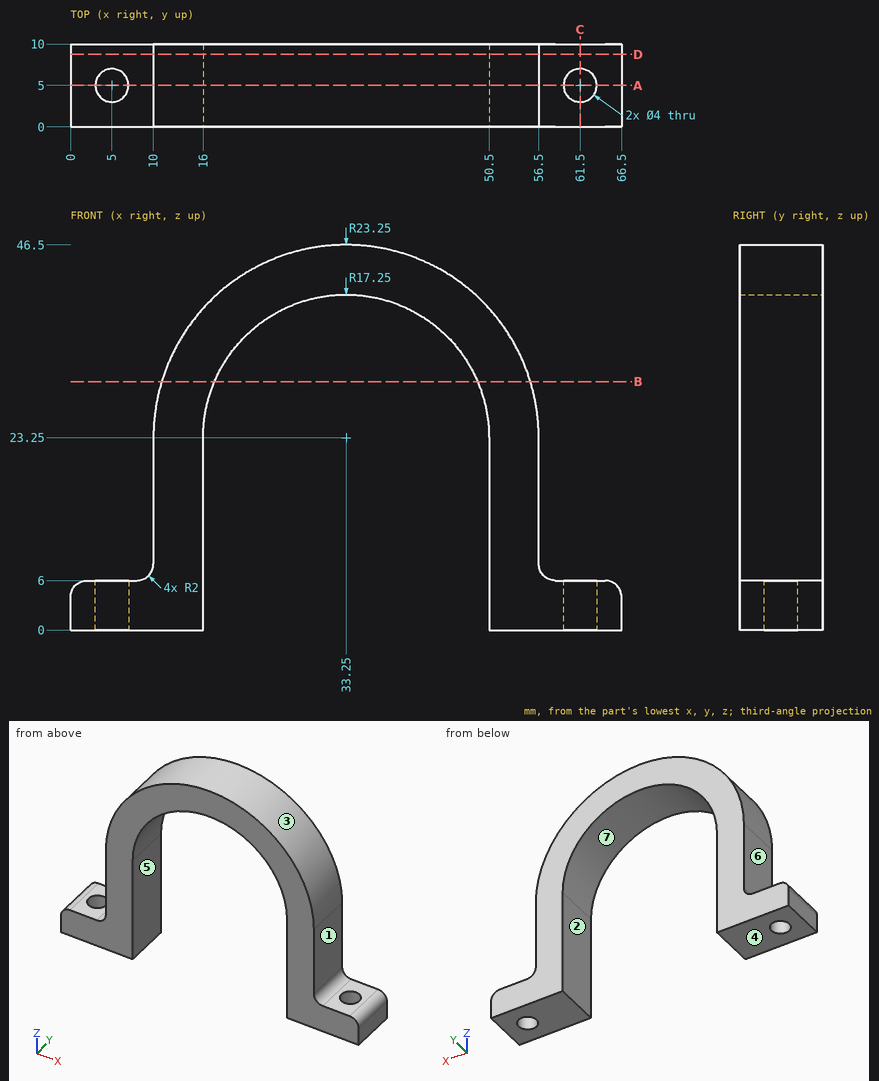
Verification items for this drawing (mm, ordinates from the low corner). A direction names the side the tool comes from. Coordinates: 2 decimals unless noted, no trailing zeros. Loops run counter-clockwise (first coordinate to the right, second up) from the corner with the lowest first, then second, coordinate; pieces in that order, holes last. Notation, with made-up numbers: (78, 15.25) - (118, 15.25) arc R12 ccw to (118, 26.25) - close; hole circle Ø5 at (3, 78.25). An arc over 180 degrees is marked (long way). Answer as a JSON object with one key per item and string values.
(1) Cross-section at A-A, the plane y = 5. Record the boundary of the cut face in (x, z), then the cut area to 3 significant figures.
Response:
{"outline": "(0, 0) - (3, 0) - (3, 6) - (2, 6) arc R2 ccw to (0, 4) - close; (7, 0) - (16, 0) - (16, 23.25) arc R17.25 cw to (50.5, 23.25) - (50.5, 0) - (59.5, 0) - (59.5, 6) - (58.5, 6) arc R2 cw to (56.5, 8) - (56.5, 23.25) arc R23.25 ccw to (10, 23.25) - (10, 8) arc R2 cw to (8, 6) - (7, 6) - close; (63.5, 0) - (66.5, 0) - (66.5, 4) arc R2 ccw to (64.5, 6) - (63.5, 6) - close", "area": "733 mm²"}
(2) Cross-section at D-D, the plane y = 8.75. Record the boundary of the cut face in (x, z).
Response:
{"outline": "(0, 0) - (16, 0) - (16, 23.25) arc R17.25 cw to (50.5, 23.25) - (50.5, 0) - (66.5, 0) - (66.5, 4) arc R2 ccw to (64.5, 6) - (58.5, 6) arc R2 cw to (56.5, 8) - (56.5, 23.25) arc R23.25 ccw to (10, 23.25) - (10, 8) arc R2 cw to (8, 6) - (2, 6) arc R2 ccw to (0, 4) - close"}
(3) Mould release check, pull along X, two halves, no side actions. Record for the marked faces 4, 5, 6 and 7: pulls with the +X half, pulls with the -X half, needs draft (parallel to the pull), parting line crosses it, or undercut.
Response:
{"face 4": "needs draft", "face 5": "undercut", "face 6": "pulls with the -X half", "face 7": "undercut"}
(4) Access from +Z, -Z, +X, -X, +Y, -Y to the whole of each face (thin tool, end or side, straight path). Record for the marked faces 1, 2 and 3.
Response:
{"face 1": "+Z, +X, +Y, -Y", "face 2": "-Z, +Y, -Y", "face 3": "+Z, +Y, -Y"}
(5) Cross-section at C-C, the plane x = 61.5. Record the boundary of the cut face in (y, z), then the cut area to 3 significant figures.
Response:
{"outline": "(0, 0) - (3, 0) - (3, 6) - (0, 6) - close; (7, 0) - (10, 0) - (10, 6) - (7, 6) - close", "area": "36.0 mm²"}
(6) Cross-section at B-B, the plane z = 30. Record the boundary of the cut face in (x, y), then the cut area to 3 significant figures.
Response:
{"outline": "(11, 0) - (17.38, 0) - (17.38, 10) - (11, 10) - close; (49.12, 0) - (55.5, 0) - (55.5, 10) - (49.12, 10) - close", "area": "127 mm²"}
(7) Go/stop test with flat-tipped pins: pin 1 Ø2 at (x, y) = (31, 6.5) entering from +Z; pin 2 Ø5 at (y, z) = (7, 16.5) entering from -X; pin 3 Ø5 at (x, y) = (5, 5) entering from +Z. Record where each tip stops, or that it passes through.
Response:
{"pin 1": "stops at z = 46.47", "pin 2": "stops at x = 10", "pin 3": "stops at z = 6"}
(8) Scan lines: line 1 along Y through (x, z) = (5, 4); line 2 along X through (y, z) = (3.5, 8.5); line 3 along Z through (x, y) = (5.5, 2). Record each from-to range of solid material in increasing order.
Response:
{"line 1": "y = 0 to 3, 7 to 10", "line 2": "x = 10 to 16, 50.5 to 56.5", "line 3": "z = 0 to 6"}
